Build history of the part. All positions in model axes, mm. A direction names the side the tool comes from. Give positions to 0.01 mm unless a question says otherwise; leave off trailing zeros. Loops run counter-clockwise (first coordinate to the right, second up) from the corner with the lowest first, then second, coordinate; pieces in that order, holes last. Notation, with made-up numbers: (57, -31) -> (76, -31) arc R16 ccw to (76, -26) -> close; hole circle Ø9 at (-1, -38.5). An arc over 180 degrees is marked (long way). One line per question, with ' | ' between items. Start each with the question number.
(1) Slice it at D-D, the plane x = 4.75. Write the cut outline in (y, z), then the cut area to 3 significant figures.
(2) Flat gauge pins, fed straight in: pin 1 Ø2 at (x, y) = (-5, 4.5) entering from -Z; pin 2 Ø1.5 at (x, z) = (3, 0) entering from +Y; pin 3 Ø6 at (y, z) = (10.5, -0.5) entering from +X; pin 4 Ø3 at (x, z) = (-3.5, -3.5) entering from +Y. Where does each tip first touch, or does it go through?
(3) Slice it at B-B, the plane y = 18.75. Write the cut outline in (x, z), then the cut area to 3 significant figures.
(4) Drill centre lines: L1, parallel to Y at x = -2, z = -5; L2, parallel to Y at x = 0.75, z = -0.5; L3, parallel to X at y = 9, z = 2.75. Where is each one in solid material? Low to high. Write a range as from..to.
(5) Slice it at A-A, the plane x = 0. Write the cut outline in (y, z).
(6) Mould opens along X. For faces 1 (the face through (3.89, 2.12, 5.3)), 2 (the face through (3, 4.3, 3)), 3 (the face through (0, 1, 1.6)) say: pulls with the +X half, pulls with the -X half, needs draft (parallel to the pull), parting line crosses it, or undercut.
(7) 3-axis set-ups, long thin cutter, end or side, ignore diameter. For faces 4 (the face through (0, 23.8, 0)), 5 (the face through (-1.15, 18.71, 2.77)), 6 (the face through (-1.38, 0.99, 0.81)): which of +Z, -Z, +X, -X, +Y, -Y reach the whole face in a straight line?
(8) Slice it at C-C, the plane y = 3. Write the cut outline in (x, z).
```python
from build123d import *

# Parameters (mm, degrees)
SKETCH_1_R          = 6.4
EXTRUDE_1_DEPTH     = 4.3
SKETCH_2_R          = 4
EXTRUDE_2_DEPTH     = 10
SKETCH_3_R          = 3
EXTRUDE_3_DEPTH     = 9.5
CUT_EXTRUDE_1_DEPTH = 2


# Read off the part's stored shape, not the designer's step: M6x1.0 机械螺纹 螺柱1
with BuildPart() as part:
    # 草图1 → 凸台-拉伸1 (new body)
    with BuildSketch(Plane(origin=(0, 0, 0), x_dir=(1, 0, 0), z_dir=(0, 1, 0))):
        with Locations(Location((0, -0.216468968, 0), (0, 0, 90))):
            Circle(SKETCH_1_R)
    extrude(amount=EXTRUDE_1_DEPTH)

    # 草图2 → 凸台-拉伸2 (add)
    with BuildSketch(Plane(origin=(0, 4.3, 0), x_dir=(1, 0, 0), z_dir=(0, 1, 0))):
        with Locations(Location((0, 0, 0), (0, 0, 270))):
            Circle(SKETCH_2_R)
    extrude(amount=EXTRUDE_2_DEPTH)

    # 草图3 → 凸台-拉伸3 (add)
    with BuildSketch(Plane(origin=(0, 14.3, 0), x_dir=(1, 0, 0), z_dir=(0, 1, 0))):
        with Locations(Location((0, 0, 0), (0, 0, 270))):
            Circle(SKETCH_3_R)
    extrude(amount=EXTRUDE_3_DEPTH)

    # M6x1.0 机械螺纹 螺柱1 outline → M6x1.0 机械螺纹 螺柱1 (revolve, cut)
    with BuildSketch(Plane.XY):
        Polygon((3, 23.8), (2.4455, 23.8), (3, 23.2455), align=None)
    revolve(axis=Axis((0, 0, 0), (0, 1, 0)), mode=Mode.SUBTRACT)

    # 草图5 → 切除-拉伸1 (cut)
    with BuildSketch(Plane.XZ):
        Polygon((1.847520861, 0), (0.923760431, 1.6), (-0.923760431, 1.6), (-1.847520861, 0), (-0.923760431, -1.6), (0.923760431, -1.6), align=None)
    extrude(amount=-CUT_EXTRUDE_1_DEPTH, mode=Mode.SUBTRACT)


solid = part.part
```
Final values:
1) outline: (0, -4.07) -> (4.3, -4.07) -> (4.3, 4.51) -> (0, 4.51) -> close | area: 36.9 mm2
2) pin 1: z = -4.76 | pin 2: y = 23.8 | pin 3: x = 4 | pin 4: y = 14.3
3) outline: circle Ø6 at (0, 0) | area: 28.3 mm2
4) L1: 0..4.3 | L2: 2..23.8 | L3: -2.9..2.9
5) outline: (0, -6.18) -> (4.3, -6.18) -> (4.3, -4) -> (14.3, -4) -> (14.3, -3) -> (23.25, -3) -> (23.8, -2.45) -> (23.8, 2.45) -> (23.25, 3) -> (14.3, 3) -> (14.3, 4) -> (4.3, 4) -> (4.3, 6.62) -> (0, 6.62) -> (0, 1.6) -> (2, 1.6) -> (2, -1.6) -> (0, -1.6) -> close
6) face 1: parting line crosses it | face 2: needs draft | face 3: undercut
7) face 4: +Z, -Z, +X, -X, +Y | face 5: +Y | face 6: -Y
8) outline: circle Ø12.8 at (0, 0.22)
